from build123d import *

# Parameters (mm, degrees)
F0_W     = 193
F0_H     = 111
F0_W_2   = 179
F0_H_2   = 97
F1_DEPTH = 2
F0_R     = 4
F0_R_2   = 2
F2_DEPTH = 4.5
F3_DEPTH = 5
F4_DEPTH = 11.85
F6_DEPTH = 50
F9_DEPTH = 25


with BuildPart() as f1:
    # F0 (on Top) → F1 (new body)
    with BuildSketch(Plane.XY):
        with Locations((38.2122632861, 15.2387920618)):
            Rectangle(F0_W, F0_H)
        with Locations((38.2122632861, 15.2387920618)):
            Rectangle(F0_W_2, F0_H_2, mode=Mode.SUBTRACT)
    extrude(amount=F1_DEPTH)

    # F0 (on Top) → F2 (join)
    with BuildSketch(Plane.XY):
        with BuildLine():
            Line((143.2122632861, 80.2387920618), (-66.7877367139, 80.2387920618))
            Line((-66.7877367139, 80.2387920618), (-66.7877367139, -49.7612079382))
            Line((-66.7877367139, -49.7612079382), (-28.393488025, -49.7612079382))
            ThreePointArc((-28.393488025, -49.7612079382), (-27.393488025, -43.1154566271), (-21.7477367139, -46.7612079382))
            ThreePointArc((-21.7477367139, -46.7612079382), (-22.1019854028, -48.4069592493), (-23.1019854028, -49.7612079382))
            Line((-23.1019854028, -49.7612079382), (104.606511975, -49.7612079382))
            ThreePointArc((104.606511975, -49.7612079382), (105.606511975, -43.1154566271), (111.2522632861, -46.7612079382))
            ThreePointArc((111.2522632861, -46.7612079382), (110.8980145972, -48.4069592493), (109.8980145972, -49.7612079382))
            Line((109.8980145972, -49.7612079382), (143.2122632861, -49.7612079382))
            Line((143.2122632861, -49.7612079382), (143.2122632861, 80.2387920618))
        make_face()
        with Locations((38.2122632861, 15.2387920618)):
            Rectangle(F0_W, F0_H, mode=Mode.SUBTRACT)
        with Locations((-25.7477367139, 75.2387920618)):
            Circle(F0_R, mode=Mode.SUBTRACT)
        with Locations((107.2522632861, 75.2387920618)):
            Circle(F0_R, mode=Mode.SUBTRACT)
        with Locations((-25.7477367139, 75.2387920618)):
            Circle(F0_R)
        with Locations((-25.7477367139, 75.2387920618)):
            Circle(F0_R_2, mode=Mode.SUBTRACT)
        with Locations((107.2522632861, 75.2387920618)):
            Circle(F0_R)
        with Locations((107.2522632861, 75.2387920618)):
            Circle(F0_R_2, mode=Mode.SUBTRACT)
        with BuildLine():
            ThreePointArc((-21.7477367139, -46.7612079382), (-27.393488025, -43.1154566271), (-28.393488025, -49.7612079382))
            Line((-28.393488025, -49.7612079382), (-23.1019854028, -49.7612079382))
            ThreePointArc((-23.1019854028, -49.7612079382), (-22.1019854028, -48.4069592493), (-21.7477367139, -46.7612079382))
        make_face()
        with Locations((-25.7477367139, -46.7612079382)):
            Circle(F0_R_2, mode=Mode.SUBTRACT)
        with BuildLine():
            Line((104.606511975, -49.7612079382), (109.8980145972, -49.7612079382))
            ThreePointArc((109.8980145972, -49.7612079382), (110.8980145972, -48.4069592493), (111.2522632861, -46.7612079382))
            ThreePointArc((111.2522632861, -46.7612079382), (105.606511975, -43.1154566271), (104.606511975, -49.7612079382))
        make_face()
        with Locations((107.2522632861, -46.7612079382)):
            Circle(F0_R_2, mode=Mode.SUBTRACT)
    extrude(amount=F2_DEPTH)

    # F0 (on Top) → F3 (cut)
    with BuildSketch(Plane.XY):
        with Locations((-25.7477367139, 75.2387920618)):
            Circle(F0_R_2)
        with Locations((107.2522632861, 75.2387920618)):
            Circle(F0_R_2)
        with Locations((107.2522632861, -46.7612079382)):
            Circle(F0_R_2)
        with Locations((-25.7477367139, -46.7612079382)):
            Circle(F0_R_2)
    extrude(amount=-F3_DEPTH, mode=Mode.SUBTRACT)

    # F0 (on Top) → F4 (join)
    with BuildSketch(Plane.XY):
        with Locations((-25.7477367139, 75.2387920618)):
            Circle(F0_R)
        with Locations((-25.7477367139, 75.2387920618)):
            Circle(F0_R_2, mode=Mode.SUBTRACT)
        with BuildLine():
            Line((104.606511975, -49.7612079382), (109.8980145972, -49.7612079382))
            ThreePointArc((109.8980145972, -49.7612079382), (110.8980145972, -48.4069592493), (111.2522632861, -46.7612079382))
            ThreePointArc((111.2522632861, -46.7612079382), (105.606511975, -43.1154566271), (104.606511975, -49.7612079382))
        make_face()
        with Locations((107.2522632861, -46.7612079382)):
            Circle(F0_R_2, mode=Mode.SUBTRACT)
        with BuildLine():
            ThreePointArc((104.606511975, -49.7612079382), (107.2522632861, -50.7612079382), (109.8980145972, -49.7612079382))
            Line((109.8980145972, -49.7612079382), (104.606511975, -49.7612079382))
        make_face()
        with BuildLine():
            ThreePointArc((-21.7477367139, -46.7612079382), (-27.393488025, -43.1154566271), (-28.393488025, -49.7612079382))
            Line((-28.393488025, -49.7612079382), (-23.1019854028, -49.7612079382))
            ThreePointArc((-23.1019854028, -49.7612079382), (-22.1019854028, -48.4069592493), (-21.7477367139, -46.7612079382))
        make_face()
        with Locations((-25.7477367139, -46.7612079382)):
            Circle(F0_R_2, mode=Mode.SUBTRACT)
        with BuildLine():
            Line((-23.1019854028, -49.7612079382), (-28.393488025, -49.7612079382))
            ThreePointArc((-28.393488025, -49.7612079382), (-25.7477367139, -50.7612079382), (-23.1019854028, -49.7612079382))
        make_face()
        with Locations((107.2522632861, 75.2387920618)):
            Circle(F0_R)
        with Locations((107.2522632861, 75.2387920618)):
            Circle(F0_R_2, mode=Mode.SUBTRACT)
    extrude(amount=F4_DEPTH)

    # F5 (on face) → F6 (join)
    with BuildSketch(Plane.XY.offset(4.5)):
        Polygon((128.084346652, 80.2387920618), (128.084346652, 70.7387920618), (134.7122632861, 70.7387920618), (143.2122632861, 70.7387920618), (143.2122632861, 80.2387920618), align=None)
        Polygon((-66.7877367139, 70.7387920618), (-58.2877367139, 70.7387920618), (-51.7344288528, 70.7387920618), (-51.7344288528, 80.2387920618), (-66.7877367139, 80.2387920618), align=None)
    extrude(amount=F6_DEPTH)

    # F8 (on face) → F9 (cut)
    with BuildSketch(Plane.XY):
        with BuildLine():
            Line((135.7841315883, 68.3924248103), (138.8478337268, 68.3924248103))
            Line((138.8478337268, 68.3924248103), (141.9115358654, 68.3924248103))
            ThreePointArc((141.9115358654, 68.3924248103), (138.8478337268, 71.4561269488), (135.7841315883, 68.3924248103))
        make_face()
        with BuildLine():
            Line((138.8478337268, 65.3287226717), (138.8478337268, 68.3924248103))
            Line((138.8478337268, 68.3924248103), (135.7841315883, 68.3924248103))
            ThreePointArc((135.7841315883, 68.3924248103), (136.6814691691, 66.2260602526), (138.8478337268, 65.3287226717))
        make_face()
        with BuildLine():
            Line((141.9115358654, 68.3924248103), (138.8478337268, 68.3924248103))
            Line((138.8478337268, 68.3924248103), (138.8478337268, 65.3287226717))
            ThreePointArc((138.8478337268, 65.3287226717), (141.0141982845, 66.2260602526), (141.9115358654, 68.3924248103))
        make_face()
        with BuildLine():
            ThreePointArc((141.8105147335, 27.6224248103), (140.9427655571, 29.7173566406), (138.8478337268, 30.5851058169))
            Line((138.8478337268, 30.5851058169), (138.8478337268, 27.6224248103))
            Line((138.8478337268, 27.6224248103), (140.926355011, 27.6224248103))
            Line((140.926355011, 27.6224248103), (141.8105147335, 27.6224248103))
        make_face()
        with BuildLine():
            Line((138.8478337268, 27.6224248103), (138.8478337268, 30.5851058169))
            ThreePointArc((138.8478337268, 30.5851058169), (136.7529018965, 25.52749298), (141.8105147335, 27.6224248103))
            Line((141.8105147335, 27.6224248103), (140.926355011, 27.6224248103))
            Line((140.926355011, 27.6224248103), (138.8478337268, 27.6224248103))
        make_face()
        with BuildLine():
            Line((-65.5505631859, 67.0167887692), (-62.4868610473, 67.0167887692))
            Line((-62.4868610473, 67.0167887692), (-59.4231589088, 67.0167887692))
            ThreePointArc((-59.4231589088, 67.0167887692), (-62.4868610473, 70.0804909077), (-65.5505631859, 67.0167887692))
        make_face()
        with BuildLine():
            Line((-62.4868610473, 63.9530866306), (-62.4868610473, 67.0167887692))
            Line((-62.4868610473, 67.0167887692), (-65.5505631859, 67.0167887692))
            ThreePointArc((-65.5505631859, 67.0167887692), (-64.653225605, 64.8504242115), (-62.4868610473, 63.9530866306))
        make_face()
        with BuildLine():
            Line((-59.4231589088, 67.0167887692), (-62.4868610473, 67.0167887692))
            Line((-62.4868610473, 67.0167887692), (-62.4868610473, 63.9530866306))
            ThreePointArc((-62.4868610473, 63.9530866306), (-60.3204964896, 64.8504242115), (-59.4231589088, 67.0167887692))
        make_face()
        with BuildLine():
            ThreePointArc((-59.5241800407, 26.2467887692), (-60.391929217, 28.3417205994), (-62.4868610473, 29.2094697758))
            Line((-62.4868610473, 29.2094697758), (-62.4868610473, 26.2467887692))
            Line((-62.4868610473, 26.2467887692), (-59.5241800407, 26.2467887692))
        make_face()
        with BuildLine():
            Line((-62.4868610473, 26.2467887692), (-62.4868610473, 29.2094697758))
            ThreePointArc((-62.4868610473, 29.2094697758), (-64.5817928776, 28.3417205994), (-65.449542054, 26.2467887692))
            Line((-65.449542054, 26.2467887692), (-62.4868610473, 26.2467887692))
        make_face()
        with BuildLine():
            Line((-59.5241800407, 26.2467887692), (-62.4868610473, 26.2467887692))
            Line((-62.4868610473, 26.2467887692), (-65.449542054, 26.2467887692))
            ThreePointArc((-65.449542054, 26.2467887692), (-62.4868610473, 23.2841077625), (-59.5241800407, 26.2467887692))
        make_face()
    extrude(amount=F9_DEPTH, mode=Mode.SUBTRACT)


solid = f1.part
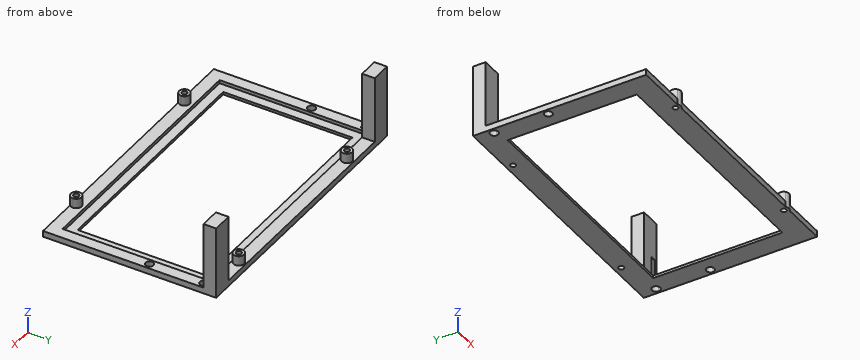
Could you check a few things on this model? Use its own coordinates, in mm. Give positions to 0.01 mm unless a question says otherwise; leave off trailing zeros. Write each loop counter-clockwise with the first axis right and the second up, starting at its lowest first coordinate (ties: lowest second). Pieces come first, ordered by that corner, then holes. Notation, with made-up numbers: (30.5, 83) -> (61.5, 83) arc R27 cw to (61.5, 109) -> close; hole circle Ø1 at (42.5, 88). An arc over 180 degrees is marked (long way). Write each question's results on one line, items separated by ' | '. Start each with the question number.
Q1. Suppose I cut it at B-B, the plane x = 3.5. List the corners of the cut face in (y, z) for me.
Q2. I'm going to push flat-ended pins straight in: pin 1 Ø2.5 at (x, y) = (-26.5, -46.5) entering from +Z; pin 2 Ø9.5 at (x, y) = (138.85, 27.62) entering from +Z; pin 3 Ø3.5 at (x, z) = (-49, 2.5) entering from -Y. Where does each tip first touch, or does it pass through?
Q3. Suppose I cut it at C-C, the plane y = 11. List the corners of the cut face in (x, z) for me.
Q4. Suppose I cut it at D-D, the plane z = 9. State how many separate pieces and enclosed holes the cut face has, and give its area (3 significant figures).
Q5. I need wall thicknesses on probe 1 along X at (y, z) = (-6, 3.5); probe 2 along Y at (x, z) = (-54.5, 36); probe 3 along Z at (x, y) = (7, 65.5). Which ranges of each line are inside material? Lowest first, please.
Q6. Suppose I cut it at A-A, the plane z = 51.5. List the corners of the cut face in (x, y) for me, and give its area (3 significant figures).
Outcome:
1) outline: (-49.76, 0) -> (-33.26, 0) -> (-33.26, 2) -> (-40.26, 2) -> (-40.26, 4.5) -> (-49.76, 4.5) -> close; (63.74, 0) -> (80.24, 0) -> (80.24, 4.5) -> (70.74, 4.5) -> (70.74, 2) -> (63.74, 2) -> close
2) pin 1: z = 11.85 | pin 2: z = 4.5 | pin 3: y = -49.76
3) outline: (-66.79, 0) -> (-51.29, 0) -> (-51.29, 2) -> (-58.29, 2) -> (-58.29, 4.5) -> (-66.79, 4.5) -> close; (127.71, 0) -> (143.21, 0) -> (143.21, 4.5) -> (134.71, 4.5) -> (134.71, 2) -> (127.71, 2) -> close
4) separate pieces: 6 | enclosed holes: 4 | area: 436 mm2
5) probe 1: -66.79 to -58.29, 134.71 to 143.21 | probe 2: 70.74 to 80.24 | probe 3: 0 to 2
6) outline: (-66.79, 70.74) -> (-51.73, 70.74) -> (-51.73, 80.24) -> (-66.79, 80.24) -> close; (128.08, 70.74) -> (143.21, 70.74) -> (143.21, 80.24) -> (128.08, 80.24) -> close | area: 287 mm2
